Part model, mm, in its own coordinate system. Face numbers are marked on the shaded views. A direction names the side the tool comes from. Round coordinates to 2 decimals unless told otherwise and drop trailing zeros. Loops run counter-clockwise (first coordinate to the right, second up) from the corner with the lowest first, then second, coordinate; pieces in that order, holes last.
from build123d import *

# Parameters (mm, degrees)
BOSS_EXTRU_1_DEPTH      = 3
BOSS_EXTRU_1_DEPTH_BACK = 3
ESQUISSE1_R             = 14.5
ESQUISSE3_R             = 1.65
ESQUISSE4_R             = 2
BOSS_EXTRU_2_DEPTH      = 2.2
CHANFREIN1_SIZE         = 0.5
ESQUISSE5_R             = 5.5
BOSS_EXTRU_3_DEPTH      = 8.8


with BuildPart() as part:
    # Esquisse1 → Boss.-Extru.1 (new, two sides: drawn at the far end of the back side and taken through both)
    with BuildSketch(Plane.XY.offset(-BOSS_EXTRU_1_DEPTH_BACK)):
        Circle(ESQUISSE1_R)
    extrude(amount=BOSS_EXTRU_1_DEPTH + BOSS_EXTRU_1_DEPTH_BACK)

    # Enl_vement de mati_re-Balayage1: sweep along a curve in space
    with BuildLine() as enl_vement_de_mati_re_balayage1_path:
        ThreePointArc((14.5, 0, 3), (10.253048327, 10.253048327, 3), (0, 14.5, 3))
        ThreePointArc((0, 14.5, 3), (-10.253048327, 10.253048327, 3), (-14.5, 0, 3))
        ThreePointArc((-14.5, 0, 3), (-10.253048327, -10.253048327, 3), (0, -14.5, 3))
        ThreePointArc((0, -14.5, 3), (10.253048327, -10.253048327, 3), (14.5, 0, 3))
    # Esquisse3 → Enl_vement de mati_re-Balayage1 (sweep, cut)
    with BuildSketch(Plane(origin=(0, 0, 0), x_dir=(0, 0, -1), z_dir=(1, 0, 0))):
        with Locations((0, 14.5)):
            Circle(ESQUISSE3_R)
    sweep(path=enl_vement_de_mati_re_balayage1_path.line, mode=Mode.SUBTRACT)

    # Esquisse4 → Boss.-Extru.2 (add)
    with BuildSketch(Plane.XY.offset(3)):
        Circle(ESQUISSE4_R)
    extrude(amount=BOSS_EXTRU_2_DEPTH)

    # Chanfrein1
    chanfrein1_edges = [part.edges().sort_by_distance(p)[0] for p in [
        (-2, 0, 5.2),
    ]]
    chamfer(chanfrein1_edges, length=CHANFREIN1_SIZE)

    # Esquisse5 → Boss.-Extru.3 (add)
    with BuildSketch(Plane(origin=(0, 0, -3), x_dir=(-1, 0, 0), z_dir=(0, 0, -1))):
        with Locations(Location((0, 0, 0), (0, 0, 180))):
            Circle(ESQUISSE5_R)
    extrude(amount=BOSS_EXTRU_3_DEPTH)


solid = part.part
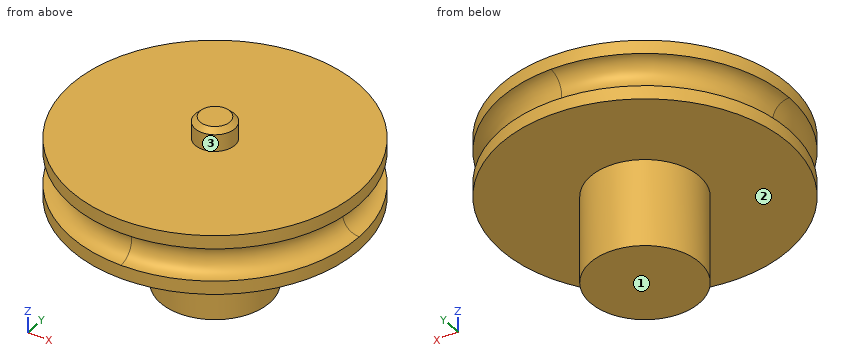
1) Slice it at B-B, the plane z = 1. Give the cut face in (x, y).
Values:
outline: circle Ø26.38 at (0, 0)
2) Slice it at A-A, the plane z = -4. Give the cut face in (x, y).
Values:
outline: circle Ø11 at (0, 0)
3) Wall check: line 1 along Z through (x, y) = (-6, 9); line 2 along Y through (x, z) = (-2, -8.25); line 3 along X through (y, z) = (5, -8). Give the ranges that are in metal, low to high.
Values:
line 1: z = -3 to 3
line 2: y = -5.12 to 5.12
line 3: x = -2.29 to 2.29
4) Tool access for the marked faces 1, 2 and 3: list every direction of +Z, -Z, +X, -X, +Y, -Y with a clear straight run to the whole face (end or side of a thin tool).
Values:
face 1: -Z, +X, -X, +Y, -Y
face 2: -Z
face 3: +Z
5) Drop flat-ended pins along their axis: pin 1 Ø4 at (x, z) = (-9, -2) entering from +Y; pin 2 Ø3 at (x, z) = (5, 0.5) entering from -Y; pin 3 Ø8.5 at (x, y) = (-5.5, 0) entering from +Z; pin 4 Ø1.5 at (y, z) = (-3.5, 0.5) entering from +X. Give the stop position or say it passes through.
Values:
pin 1: stops at y = 12.7
pin 2: stops at y = -13.93
pin 3: stops at z = 5.2
pin 4: stops at x = 12.98
